Autodesk Inventor part; units mm, degrees
ref_plane "Work Plane1" through (0, 0, -17.54) normal (0, 0, 1) x (1, 0, 0)
ref_plane "YZ Plane" through (0, 0, 0) normal (1, 0, 0) x (0, 1, 0)
ref_plane "XZ Plane" through (0, 0, 0) normal (0, 1, 0) x (-1, 0, 0)
sketch "Sketch1" plane through (0, 0, 0) normal (0, 0, 1) x (1, 0, 0)
  line L0 (12.54, 0) -> (22.54, 0)
  line L1 (22.54, 0) -> (22.54, 3)
  line L2 (22.54, 3) -> (12.54, 3)
  line L3 (12.54, 3) -> (12.54, 0)
  line L4 (12.54, 0) -> (17.54, 0)
  line L5 (17.54, 0) -> (17.54, -5)
  line L6 (17.54, -5) -> (12.54, -5)
  line L7 (12.54, -5) -> (12.54, 0)
  line L8 (0, -6.6) -> (0, 4.6)
  point P0 (0, 0)
  point P1 (17.54, 0)
  dimension "d0" = 3
  dimension "d1" = 12.54
  dimension "d2" = 10
  dimension "d3" = 5
  dimension "d4" = 5
revolve "Revolution1" add sketch "Sketch1" angle 360 about axis through (0, -10, 0) along (0, 1, 0)
sketch "Sketch2" plane through (0, 0, 0) normal (0, 0, 1) x (1, 0, 0)
  line L0 (12.54, -5) -> (-12.54, -5)
  line L1 (12.54, 3) -> (-12.54, 3)
  line L2 (0, 0) -> (0, -5) construction
  point P0 (0, -2.5)
hole "Hole1" at (0, -2.5, 0) direction (0, 0, -1) diameter 3.4 end through all
chamfer "Chamfer1" distance 0.5 angle 45 2 edges at (-12.54, -5, 0) (-12.54, 3, 0)
ref_plane "Work Plane1" through (0, 0, -17.54) normal (0, 0, 1) x (1, 0, 0)
sketch "Sketch3" plane through (0, 0, -17.54) normal (0, 0, 1) x (1, 0, 0)
  line L0 (-0.5, -0.8752) -> (0.5, -0.8752)
  line L1 (0.5, -0.8752) -> (0.5, -4.1248)
  line L2 (0.5, -4.1248) -> (-0.5, -4.1248)
  line L3 (-0.5, -4.1248) -> (-0.5, -0.8752)
  line L4 (-0.5, -0.8752) -> (0.5, -4.1248) construction
  line L5 (0.5, -0.8752) -> (-0.5, -4.1248) construction
  line L6 (0.5, -4.1248) -> (-0.5, -4.1248)
  line L7 (-0.5, -4.1248) -> (-0.5, -4.3248)
  line L8 (-0.5, -4.3248) -> (0.5, -4.3248)
  line L9 (0.5, -4.3248) -> (0.5, -4.1248)
  line L10 (0.5, -0.8752) -> (-0.5, -0.8752)
  line L11 (-0.5, -0.8752) -> (-0.5, -0.6752)
  line L12 (-0.5, -0.6752) -> (0.5, -0.6752)
  line L13 (0.5, -0.6752) -> (0.5, -0.8752)
  point P0 (0, 0)
  point P1 (1.7, -2.5)
  point P2 (1.7, -2.5)
  point P3 (1.7, -2.5)
  point P4 (0, -2.5)
  dimension "d22" = 1
  dimension "d24" = 0.2
  dimension "d25" = 0.2
extrude "Extrusion1" cut sketch "Sketch3" along normal blind 20 contours L11 L12 L13 L0 | L2 L9 L8 L7
properties part number "spring safety  for print"
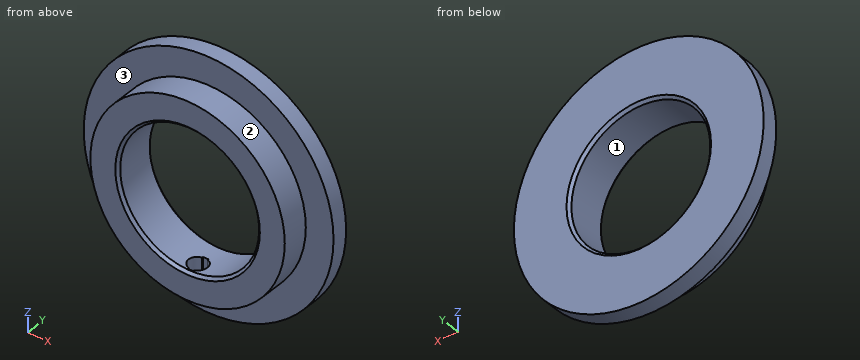
Build history of the part. All positions in model axes, mm. Face numbers are marked on the shaded views. Round coordinates to 2 decimals unless told otherwise and drop trailing zeros. Write each loop counter-clockwise with the first axis right and the second up, starting at its lowest first coordinate (ties: lowest second). Pieces come first, ordered by that corner, then holes. Notation, with made-up numbers: (42, 17.5) -> (48, 17.5) arc R7 cw to (48, 26.5) -> close; hole circle Ø10 at (73.25, 50.5). An arc over 180 degrees is marked (long way). Put each result on its own line as item: value.
Item 1: Slice it at A-A, the plane z = 0. Give the cut face in (x, y), plus the area to 4 significant figures.
Here are the results:
outline: (-22.54, 0) -> (-17.54, 0) -> (-17.54, -5) -> (-13.04, -5) -> (-12.54, -4.5) -> (-12.54, 2.5) -> (-13.04, 3) -> (-22.54, 3) -> close; (12.54, -4.5) -> (13.04, -5) -> (17.54, -5) -> (17.54, 0) -> (22.54, 0) -> (22.54, 3) -> (13.04, 3) -> (12.54, 2.5) -> close
area: 109.5 mm^2
Item 2: Wall check: probe 1 along X at (y, z) = (-0.25, -0.5); probe 2 along X at (y, z) = (0.5, 0). Give the ranges that are in metal, low to high. Write a range as from..to.
Here are the results:
probe 1: x = -17.53..-12.53, 12.53..17.53
probe 2: x = -22.54..-12.54, 12.54..22.54
Item 3: Two-plate mould, pull along X, no slides. Class the marked faces 1, 2 and 3: pulls with the +X half, pulls with the -X half, needs draft (parallel to the pull), parting line crosses it, or undercut.
Here are the results:
face 1: undercut
face 2: parting line crosses it
face 3: needs draft
Item 4: Slice it at B-B, the plane y = -2. Give the cut face in (x, z).
Here are the results:
outline: (-1.62, -17.46) -> (-1.62, -12.43) arc R12.54 cw (long way) to (1.62, -12.43) -> (1.62, -17.46) arc R17.54 ccw (long way) to start
Item 5: Flat gauge pins, fed straight in: P1, Ø3, axis at x = 2, y = 0, coming from the -Z side; P2, Ø4, axis at y = -2.5, z = -17, coming from the -X side; P3, Ø20, axis at x = 0, z = 0, coming from the +Y side. Where does each tip first touch, or does it go through?
Here are the results:
P1: stops at z = -22.53
P2: stops at x = -9.09
P3: passes through
